```python
from build123d import *

# Parameters (mm, degrees)
SKETCH1_W           = 25.4
SKETCH1_H           = 25.4
SKETCH1_W_2         = 22.225
SKETCH1_H_2         = 22.225
BOSS_EXTRUDE1_DEPTH = 152.4
CUT_EXTRUDE1_DEPTH  = 156.02325632


with BuildPart() as part:
    # Sketch1 → Boss-Extrude1 (new body)
    with BuildSketch(Plane.XY):
        Rectangle(SKETCH1_W, SKETCH1_H)
        Rectangle(SKETCH1_W_2, SKETCH1_H_2, mode=Mode.SUBTRACT)
    extrude(amount=BOSS_EXTRUDE1_DEPTH)

    # Sketch2 → Cut-Extrude1 (cut, through all)
    with BuildSketch(Plane(origin=(0, 12.7, 0), x_dir=(1, 0, 0), z_dir=(0, 1, 0))):
        with BuildLine():
            Line((-12.7, 0), (12.7, 0))
            ThreePointArc((12.7, 0), (0, -5.821345112), (-12.7, 0))
        make_face()
        with BuildLine():
            Line((12.7, -152.4), (-12.7, -152.4))
            ThreePointArc((-12.7, -152.4), (0, -146.578654888), (12.7, -152.4))
        make_face()
    extrude(amount=-CUT_EXTRUDE1_DEPTH, mode=Mode.SUBTRACT)


solid = part.part
```
The listing builds one solid part. Answer for the finished solid, in the listing's coordinates (mm). A direction names the side the tool comes from. Round coordinates to 2 decimals unless told otherwise and drop trailing zeros. Write each loop counter-clockwise with the first axis right and the second up, starting at its lowest first coordinate (ties: lowest second). Pieces come first, ordered by that corner, then holes. Notation, with made-up numbers: (63, -18) -> (72, -18) arc R27 ccw to (72, 14) -> close; hole circle Ø11 at (-6, 18.5). An arc over 180 degrees is marked (long way). Answer as a JSON object with one key per item and string values. Group by question number.
Q1. Which of the six approach directions +Z, -Z, +X, -X, +Y, -Y give full straight-line access (tool end or side, diameter ignored) to faces 4 (the face through (12.7, 0, 75)), 5 (the face through (-11.112, 0, 75))?
Q2. Each of these flat-tipped pins is pushed along its axis until it touches: pin 1 Ø4 at (x, y) = (-6.5, 8) entering from +Z; pin 2 Ø12 at (x, y) = (1.5, 5.5) entering from +Z; pin 3 Ø10 at (x, y) = (6.5, -10) entering from -Z. Where does it stop, or does it pass through?
Q3. Determine the mould class of faces 1 (the face through (0, -12.7, 75)), 2 (the face through (11.112, 0, 75)), 3 (the face through (0, 12.7, 75)) for opening direction Y: pulls with the +Y half, pulls with the -Y half, needs draft (parallel to the pull), parting line crosses it, or undercut.
Q4. Section A-A (y = -8) is taken. Write down the section's boundary in (x, z).
Q5. Section B-B (z = 44) is taken. Write down the section's boundary in (x, y), plus the area to 3 significant figures.
Q6. A straight line is drawn through the part: line 1 along X through (y, z) = (-0.75, 23). Find the intervals that lie inside material, in ascending order.
Q7. Section C-C (x = 5.5) is taken. Write down the section's boundary in (y, z), plus the area to 3 significant figures.
Check values:
{
 "1": {"face 4": "+Z, -Z, +X, +Y, -Y", "face 5": "+Z, -Z"},
 "2": {"pin 1": "through", "pin 2": "z = 146.97", "pin 3": "z = 1.25"},
 "3": {"face 1": "pulls with the -Y half", "face 2": "undercut", "face 3": "pulls with the +Y half"},
 "4": {"outline": "(-12.7, 0) arc R16.76 cw to (-11.11, 1.61) -> (-11.11, 150.79) arc R16.76 cw to (-12.7, 152.4) -> close; (11.11, 1.61) arc R16.76 cw to (12.7, 0) -> (12.7, 152.4) arc R16.76 cw to (11.11, 150.79) -> close"},
 "5": {"outline": "(-12.7, -12.7) -> (12.7, -12.7) -> (12.7, 12.7) -> (-12.7, 12.7) -> close; hole (-11.11, -11.11) -> (11.11, -11.11) -> (11.11, 11.11) -> (-11.11, 11.11) -> close", "area": "151 mm^2"},
 "6": {"line 1": "-12.7 to -11.11, 11.11 to 12.7"},
 "7": {"outline": "(-12.7, 4.89) -> (-11.11, 4.89) -> (-11.11, 147.51) -> (-12.7, 147.51) -> close; (11.11, 4.89) -> (12.7, 4.89) -> (12.7, 147.51) -> (11.11, 147.51) -> close", "area": "453 mm^2"}
}
